Autodesk Fusion 360 part; units mm, degrees
sketch "Sketch1" plane through (0, 0, 0) normal (1, 0, 0) x (0, 1, 0)
  line L0 (-70, 0) -> (110, 0)
  line L1 (0, 110) -> (0, -170)
  line L2 (-15.2069, 0) -> (-20, 0)
  line L3 (-20, 0) -> (-20, -82.5)
  line L4 (-20, -82.5) -> (55, -82.5)
  line L5 (55, -82.5) -> (55, -47.4706)
  line L6 (51.4853, -38.9853) -> (13.3243, -0.8243)
  line L7 (55, -42.5) -> (115.1063, -42.5) construction
  arc A0 (12.4562, 1.046) -> (-12.2636, 2.4194) centre (0, 0) ccw
  arc A1 (-15.2069, 0) -> (-12.2636, 2.4194) centre (-15.2069, 3) ccw
  arc A2 (12.4562, 1.046) -> (13.3243, -0.8243) centre (15.4456, 1.297) ccw
  arc A3 (55, -47.4706) -> (51.4853, -38.9853) centre (43, -47.4706) ccw
  point P0 (-12.5, 0)
  dimension "d2" = 7.5
  dimension "d3" = 82.5
  dimension "d4" = 75
  dimension "d5" = 40
  dimension "d6" = 135
  dimension "d7" = 12.5
  dimension "d8" = 3
  dimension "d9" = 3
  dimension "d10" = 12
extrude "Extrude1" add sketch "Sketch1" along normal blind 65
sketch "Sketch2" plane through (65, 0, 0) normal (1, 0, 0) x (0, 1, 0)
  line L0 (-15.2069, 0) -> (-20, 0)
  line L1 (-20, 0) -> (-20, -82.5)
  line L2 (-20, -82.5) -> (55, -82.5)
  line L3 (55, -82.5) -> (55, -47.4706)
  arc A0 (55, -47.4706) -> (51.4853, -38.9853) centre (43, -47.4706) ccw
  line L4 (51.4853, -38.9853) -> (13.3243, -0.8243)
  arc A1 (12.4562, 1.046) -> (13.3243, -0.8243) centre (15.4456, 1.297) ccw
  arc A2 (12.4562, 1.046) -> (-12.2636, 2.4194) centre (0, 0) ccw
  arc A3 (-15.2069, 0) -> (-12.2636, 2.4194) centre (-15.2069, 3) ccw
sketch "Sketch3" plane through (0, -20, 0) normal (0, -1, 0) x (1, 0, 0)
  line L0 (0, 0) -> (0, -82.5)
  line L1 (0, -82.5) -> (65, -82.5)
  line L2 (65, -82.5) -> (65, 0)
  line L3 (65, 0) -> (0, 0)
  line L4 (0, 0) -> (32.5, 0)
  line L5 (32.5, 0) -> (32.5, -42.5)
  circle A0 centre (32.5, -42.5) radius 22.5
  dimension "d13" = 42.5
  dimension "d14" = 45
extrude "Extrude2" cut sketch "Sketch3" against normal blind 110 contours A0
sketch "Sketch4" plane through (0, -20, 0) normal (0, -1, 0) x (1, 0, 0)
  circle A0 centre (32.5, -42.5) radius 22.5
  line L0 (0, 0) -> (0, -82.5)
  line L1 (0, -82.5) -> (65, -82.5)
  line L2 (65, -82.5) -> (65, 0)
  line L3 (65, 0) -> (0, 0)
  circle A1 centre (32.5, -42.5) radius 40
  dimension "d17" = 80
extrude "Extrude3" cut sketch "Sketch4" against normal blind 110 contours L0 L1 A1 | L1 L2 A1
sketch "Sketch5" plane through (0, 0, 0) normal (0, 1, 0) x (1, 0, 0)
sketch "Sketch6" plane through (65, 0, 0) normal (1, 0, 0) x (0, 1, 0)
  circle A0 centre (0, 0) radius 4.5
  dimension "d23" = 9
extrude "Extrude4" cut sketch "Sketch6" against normal blind 120
sketch "Sketch7" plane through (65, 17.5, -34.7081) normal (1, 0, 0) x (0, 1, 0)
sketch "Sketch8" plane through (0, 0, 0) normal (-1, 0, 0) x (0, -1, 0)
  circle A0 centre (0, 0) radius 4.5
  line L0 (-55, -65.8184) -> (20, -65.8184)
  line L1 (20, -65.8184) -> (20, 0)
  line L2 (20, 0) -> (15.2069, 0)
  arc A1 (12.2636, 2.4194) -> (15.2069, 0) centre (15.2069, 3) ccw
  arc A2 (12.2636, 2.4194) -> (-12.4562, 1.046) centre (0, 0) ccw
  arc A3 (-13.3243, -0.8243) -> (-12.4562, 1.046) centre (-15.4456, 1.297) ccw
  line L3 (-13.3243, -0.8243) -> (-51.4853, -38.9853)
  arc A4 (-51.4853, -38.9853) -> (-55, -47.4706) centre (-43, -47.4706) ccw
  line L4 (-55, -47.4706) -> (-55, -65.8184)
  circle A5 centre (0, 0) radius 7.5
  dimension "d26" = 15
extrude "Extrude5" cut sketch "Sketch8" against normal blind 8 contours A5
sketch "Sketch9" plane through (0, -20, 0) normal (0, -1, 0) x (1, 0, 0)
  circle A0 centre (32.5, -42.5) radius 22.5
  arc A1 (0, -65.8184) -> (65, -65.8184) centre (32.5, -42.5) ccw
  line L0 (65, -65.8184) -> (65, 0)
  line L1 (65, 0) -> (0, 0)
  line L2 (0, 0) -> (0, -65.8184)
  line L3 (31, -42.5) -> (34, -42.5)
  line L4 (34, -42.5) -> (34, 31.8842)
  line L5 (34, 31.8842) -> (31, 31.8842)
  line L6 (31, 31.8842) -> (31, -42.5)
  dimension "d30" = 3
extrude "Extrude6" cut sketch "Sketch9" against normal blind 130 contours A0 L3 L4 L6 | A0 L1 L4 L6 | L1 L4 L5 L6 picked at (31.959, -57.4579)
Geometry check sheet. Reference: the model listing, model coordinates, mm. A direction names the side the tool comes from. Give positions to 0.01 mm unless a question says otherwise; leave off trailing zeros. Loops run counter-clockwise (first coordinate to the right, second up) from the corner with the lowest first, then second, coordinate; pieces in that order, holes last. Notation, with made-up numbers: (70, 55.25) -> (104, 55.25) arc R7 cw to (104, 61.25) -> close; hole circle Ø7 at (29.5, 74.5). An arc over 180 degrees is marked (long way). Answer in a Markdown table with one row per item. Add a question column.
1) Cross-section at A-A on z = -14.5. Record the boundary of the cut face in (x, y).
2) Draft check along X on faces 6 (the face through (31.53, 16.98, -64.98)), 7 (the face through (31.969, 16.975, -82.496)), 8 (the face through (15.283, 0.443, 12.492)). Enter one of: pulls with the +X half, pulls with the -X half, needs draft (parallel to the pull), parting line crosses it, or undercut.
3) Cross-section at D-D on y = 16.5. Record the boundary of the cut face in (x, z), and give its area (3 significant figures).
4) Set-up check for faces 1 (the face through (8, 0, -5)), 2 (the face through (11.8, 28.4, -15.9)), 3 (the face through (49, -18, 0)), 4 (the face through (31, 0, -7)), 5 (the face through (32, 55, -65.2)): record each of +Z, -Z, +X, -X, +Y, -Y from which the full face is reachable in a straight line by a thin tool's end or side.
5) Material ranges on probe 1 along Z at (x, y) = (42.5, 0); probe 2 along Z at (x, y) = (36.5, 0.5); probe 3 along X at (y, z) = (10.5, -5), recorded low to high. Write a range as from..to.
6) Cross-section at C-C on x = 17.5. Record the boundary of the cut face in (y, z), and give its area (3 significant figures).
7) Cross-section at B-B on y = 0. Record the boundary of the cut face in (x, z).
8) Gauge pin test, flat ends, axial feed: P1, Ø7.5, axis at y = -1.5, z = -2, coming from the -X side; P2, Ø12, axis at x = 30.5, z = -53, coming from the -Y side; P3, Ø5.5, axis at x = 19.5, y = -17.5, coming from the +Z side (3 decimals); P4, Ø4, axis at x = 28, y = 18.5, coming from the +Z side. Record the tip position at first contact, or that the pin passes through.
Outcome:
| question | item | result |
|---|---|---|
| 1 | outline | (0, -20) -> (31, -20) -> (31, 27) -> (0, 27) -> close; (34, -20) -> (65, -20) -> (65, 27) -> (34, 27) -> close |
| 2 | face 6 | undercut |
| 2 | face 7 | parting line crosses it |
| 2 | face 8 | needs draft |
| 3 | outline | (0, -65.82) arc R40 ccw to (65, -65.82) -> (65, -4) -> (34, -4) -> (34, -20.05) arc R22.5 cw (long way) to (31, -20.05) -> (31, -4) -> (0, -4) -> close |
| 3 | area | 3,140 mm^2 |
| 4 | face 1 | -X |
| 4 | face 2 | +Z, +X, -X, +Y |
| 4 | face 3 | +Z, +X, -X, -Y |
| 4 | face 4 | +Z, +Y, -Y |
| 4 | face 5 | +Z, -Z, +X, -X, +Y |
| 5 | probe 1 | z = -81.23..-62.66, -22.34..-4.5, 4.5..12.5 |
| 5 | probe 2 | z = -82.3..-64.64, -20.36..-4.47, 4.47..12.49 |
| 5 | probe 3 | x = 0..31, 34..65 |
| 6 | outline | (-20, -79.58) -> (55, -79.58) -> (55, -59.27) -> (-20, -59.27) -> close; (-20, -25.73) -> (38.23, -25.73) -> (13.32, -0.82) arc R3 cw to (12.46, 1.05) arc R12.5 ccw to (-12.26, 2.42) arc R3 cw to (-15.21, 0) -> (-20, 0) -> close; hole circle Ø9 at (0, 0) |
| 6 | area | 2,870 mm^2 |
| 7 | outline | (0, -65.82) arc R40 ccw to (65, -65.82) -> (65, -4.5) -> (34, -4.5) -> (34, -20.05) arc R22.5 cw (long way) to (31, -20.05) -> (31, -4.5) -> (8, -4.5) -> (8, -7.5) -> (0, -7.5) -> close; (0, 7.5) -> (8, 7.5) -> (8, 4.5) -> (31, 4.5) -> (31, 12.5) -> (0, 12.5) -> close; (34, 4.5) -> (65, 4.5) -> (65, 12.5) -> (34, 12.5) -> close |
| 8 | P1 | stops at x = 8 |
| 8 | P2 | passes through |
| 8 | P3 | stops at z = 0.035 |
| 8 | P4 | stops at z = -4 |
